Part print with two shaded views. Sizes in mm from the minimum x, y, z corner. Round coordinates to 2 decimals unless told otherwise and drop trailing zeros. Loops run counter-clockwise (first coordinate to the right, second up) from the corner with the lowest first, then second, coordinate; pieces in that order, holes last. Notation, with made-up numbers: (30.25, 15.25) -> (65.25, 15.25) arc R22 ccw to (65.25, 54.25) -> close; hole circle Ø10 at (12.25, 74). An arc over 180 degrees is marked (long way). Put each result on its own line as item: value. Start each with the question number.
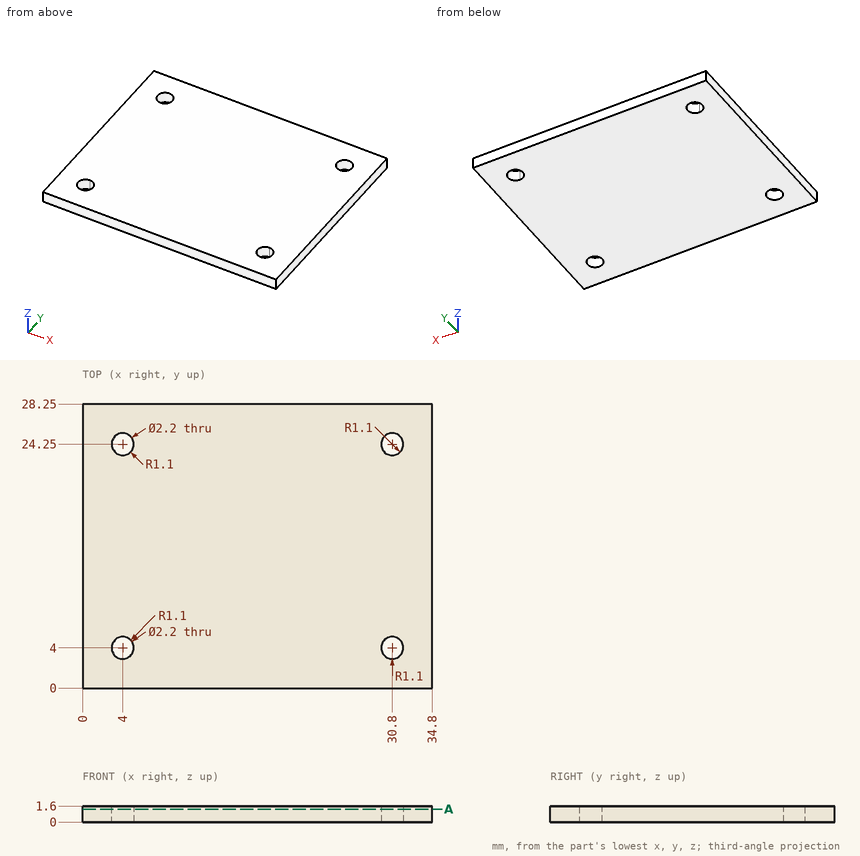
Item 1: Wall check: line 1 (Y direction, x = 4, z = 1.05); line 2 (X direction, y = 4, z = 1.1); line 3 (Y direction, x = 4.5, z = 1.5). Give the ranges that are in metal, low to high. Write a range as from..to.
Item 2: Cut at A-A on z = 1.3. Write the cut outline in (x, y).
Item 3: Drop a flat-ended pin along its axis: pin 1 (1.3 mm diameter, centred on x = 4, y = 4, fed in from -Z). Give the stop position or say it passes through.
Ans:
1. line 1: y = 0..2.9, 5.1..23.15, 25.35..28.25
1. line 2: x = 0..2.9, 5.1..29.7, 31.9..34.8
1. line 3: y = 0..3.02, 4.98..23.27, 25.23..28.25
2. outline: (0, 0) -> (34.8, 0) -> (34.8, 28.25) -> (0, 28.25) -> close; hole (4, 5.1) arc R1.1 ccw (long way) to (5.1, 4) arc R1.1 ccw to start; hole (4, 23.15) arc R1.1 ccw to (5.1, 24.25) arc R1.1 ccw (long way) to start; hole (29.7, 4) arc R1.1 ccw to (31.9, 4) arc R1.1 ccw to (30.8, 5.1) arc R1.1 ccw to start; hole (29.7, 24.25) arc R1.1 ccw to (30.8, 23.15) arc R1.1 ccw to (31.9, 24.25) arc R1.1 ccw to start
3. pin 1: passes through
